Here's how the part is built. I have some questions about the finished solid (model axes, mm). Round coordinates to 2 decimals unless told otherwise and drop trailing zeros. Loops run counter-clockwise (first coordinate to the right, second up) from the corner with the lowest first, then second, coordinate; pieces in that order, holes last. Notation, with made-up numbers: M 75.25,-16.75 L 129.25,-16.75 A24 cw 129.25,-5.75 Z; hole C 73.25,-2.5 d9. An arc over 180 degrees is marked long. Answer as a JSON object with one key per item and string values.
from build123d import *

# Parameters (mm, degrees)
F0_R     = 1.5
F0_W     = 17.4
F0_H     = 17.4
F1_DEPTH = 6
F2_R     = 0.8
F3_R     = 1


with BuildPart() as f1:
    # F0 (on Top) → F1 (new body)
    with BuildSketch(Plane.XY):
        Polygon((0, 21), (0, 0), (66, 0), (66, 77), (51, 77), align=None)
        with Locations((4, 4.5)):
            Circle(F0_R, mode=Mode.SUBTRACT)
        with Locations((16, 18.5)):
            Rectangle(F0_W, F0_H, mode=Mode.SUBTRACT)
        with Locations((35, 18.5)):
            Rectangle(F0_W, F0_H, mode=Mode.SUBTRACT)
        with Locations((62, 4.5)):
            Circle(F0_R, mode=Mode.SUBTRACT)
        with Locations((54, 18.5)):
            Rectangle(F0_W, F0_H, mode=Mode.SUBTRACT)
        with Locations((35, 37.5)):
            Rectangle(F0_W, F0_H, mode=Mode.SUBTRACT)
        with Locations((54, 37.5)):
            Rectangle(F0_W, F0_H, mode=Mode.SUBTRACT)
        with Locations((54, 56.5)):
            Rectangle(F0_W, F0_H, mode=Mode.SUBTRACT)
        with Locations((57, 72.5)):
            Circle(F0_R, mode=Mode.SUBTRACT)
    extrude(amount=F1_DEPTH)

    # F2
    f2_edges = [f1.edges().sort_by_distance(p)[0] for p in [
        (7.3, 27.2, 3),
        (26.3, 27.2, 3),
        (45.3, 27.2, 3),
        (26.3, 46.2, 3),
        (45.3, 46.2, 3),
        (45.3, 65.2, 3),
        (62.7, 65.2, 3),
        (62.7, 46.2, 3),
        (62.7, 27.2, 3),
        (43.7, 46.2, 3),
        (43.7, 27.2, 3),
        (24.7, 27.2, 3),
        (62.7, 47.8, 3),
        (62.7, 28.8, 3),
        (62.7, 9.8, 3),
        (43.7, 9.8, 3),
        (24.7, 9.8, 3),
        (43.7, 28.8, 3),
        (26.3, 28.8, 3),
        (26.3, 9.8, 3),
        (7.3, 9.8, 3),
        (45.3, 9.8, 3),
        (45.3, 28.8, 3),
        (45.3, 47.8, 3),
    ]]
    fillet(f2_edges, radius=F2_R)

    # F3
    f3_edges = [f1.edges().sort_by_distance(p)[0] for p in [
        (66, 77, 3),
        (51, 77, 3),
        (0, 21, 3),
        (0, 0, 3),
        (66, 0, 3),
    ]]
    fillet(f3_edges, radius=F3_R)


solid = f1.part
Item 1: Please list where these lines run through material, in increasing order: probe 1 along Y at (x, z) = (57, 3.75); probe 2 along Y at (x, z) = (48.5, 5.65); probe 3 along X at (y, z) = (27, 4.55). Write a range as from..to.
Resolved:
{"probe 1": "0..9.8, 27.2..28.8, 46.2..47.8, 65.2..71, 74..77", "probe 2": "0..9.8, 27.2..28.8, 46.2..47.8, 65.2..74.25", "probe 3": "5.46..7.57, 24.43..26.57, 43.43..45.57, 62.43..66"}
Item 2: If we mould it in two halves opening along Y, with no side actions, what happens to faces 1 (the face through (25.835, 49.367, 2.958)), 2 (the face through (54, 47.8, 3)), 3 (the face through (33, 0, 3)), 4 (the face through (43.7, 18, 3))? For each: pulls with the +Y half, pulls with the -Y half, needs draft (parallel to the pull), parting line crosses it, or undercut.
Resolved:
{"face 1": "pulls with the +Y half", "face 2": "undercut", "face 3": "pulls with the -Y half", "face 4": "undercut"}
Item 3: I'm going to push flat-ended pins straight in: pin 1 Ø12 at (x, y) = (28, 65) entering from +Z; pin 2 Ø3.5 at (x, y) = (57, 72.5) entering from +Z; pin 3 Ø1.8 at (y, z) = (35.5, 3.5) entering from -X; pin 4 Ø1.8 at (x, z) = (15, 2.5) entering from +Y. Where does each tip first touch, or does it pass through?
Resolved:
{"pin 1": "through", "pin 2": "z = 6", "pin 3": "x = 12.39", "pin 4": "y = 38.46"}
Item 4: I want a section at B-B, the plane y = 4.5. Please give me the cut outline in (x, z), then the cut area to 3 significant figures.
Resolved:
{"outline": "M 0,0 L 2.5,0 L 2.5,6 L 0,6 Z; M 5.5,0 L 60.5,0 L 60.5,6 L 5.5,6 Z; M 63.5,0 L 66,0 L 66,6 L 63.5,6 Z", "area": "360 mm²"}
Item 5: I want a section at D-D, the plane y = 59. Please give me the cut outline in (x, z).
Resolved:
{"outline": "M 34.61,0 L 45.3,0 L 45.3,6 L 34.61,6 Z; M 62.7,0 L 66,0 L 66,6 L 62.7,6 Z"}
Item 6: I want a section at A-A, the plane x = 57. Please give me the cut outline in (y, z), then the cut area to 3 significant figures.
Resolved:
{"outline": "M 0,0 L 9.8,0 L 9.8,6 L 0,6 Z; M 27.2,0 L 28.8,0 L 28.8,6 L 27.2,6 Z; M 46.2,0 L 47.8,0 L 47.8,6 L 46.2,6 Z; M 65.2,0 L 71,0 L 71,6 L 65.2,6 Z; M 74,0 L 77,0 L 77,6 L 74,6 Z", "area": "131 mm²"}
Item 7: I want a section at C-C, the plane y = 15. Please give me the cut outline in (x, z).
Resolved:
{"outline": "M 0,0 L 7.3,0 L 7.3,6 L 0,6 Z; M 24.7,0 L 26.3,0 L 26.3,6 L 24.7,6 Z; M 43.7,0 L 45.3,0 L 45.3,6 L 43.7,6 Z; M 62.7,0 L 66,0 L 66,6 L 62.7,6 Z"}
